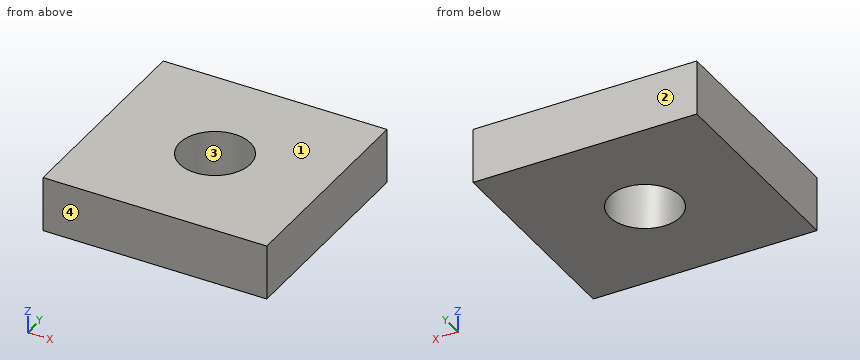
```python
from build123d import *

# Parameters (mm, degrees)
F0_R     = 16.2815755653
F1_DEPTH = 25.4
F3_DEPTH = 25.4


# Not quite as in the source:
# - the program builds the solid bodies; features that only make, move or delete a surface that nothing else refers to are left out


with BuildPart() as f1:
    # F0 (on Top) → F1 (new body)
    with BuildSketch(Plane.XY):
        Polygon((-32.1844741702, 49.3294708431), (-51.5748507939, 49.3294708431), (-51.5748507939, -49.3294708431), (51.5748507939, -49.3294708431), (51.5748507939, 49.3294708431), (-11.7852937953, 49.3294708431), align=None)
        Circle(F0_R, mode=Mode.SUBTRACT)
    extrude(amount=F1_DEPTH)

    # F0 (on Top) → F3 (join)
    with BuildSketch(Plane.XY):
        Polygon((-32.1844741702, 49.3294708431), (-51.5748507939, 49.3294708431), (-51.5748507939, -49.3294708431), (51.5748507939, -49.3294708431), (51.5748507939, 49.3294708431), (-11.7852937953, 49.3294708431), align=None)
        Circle(F0_R, mode=Mode.SUBTRACT)
    extrude(amount=F3_DEPTH)


solid = f1.part
```
The model under review builds one solid part; all positions refer to its coordinate system, in mm. Face numbers are marked on the shaded views. Round coordinates to 2 decimals unless told otherwise and drop trailing zeros. Order: outer loops, then holes, each group sorted by start corner. A loop starts at its lowest first (then second) coordinate and runs counter-clockwise, first axis right, second up. Notation, with made-up numbers: (48, 36.25) -> (104, 36.25) arc R32 ccw to (104, 64.25) -> close; hole circle Ø9 at (46.25, 38). An arc over 180 degrees is marked (long way). One line per item, written item: value. Start each with the question number.
Q1. Wall thickness on line 1 (Y direction, x = 0, z = 10); line 2 (Y direction, x = 3, z = 10.25): over which ranges is each line inside the solid? List them lowest first.
Q2. Take a section at B-B (x = 0). Write out the cut boundary in (y, z), and give its area (3 significant figures).
Q3. Take a section at C-C (z = 22.5). Write out the cut boundary in (x, y), and give its area (3 significant figures).
Q4. Take a section at A-A (y = 0). Write out the cut boundary in (x, z), and give its area (3 significant figures).
Q5. Mouldability with a two-part tool opening along Y and no side actions: class the marked faces 1, 2, 3 and 4 as released by +Y, released by -Y, zero draft, split by the parting line, or undercut.
Reported:
1. line 1: y = -49.33 to -16.28, 16.28 to 49.33
1. line 2: y = -49.33 to -16, 16 to 49.33
2. outline: (-49.33, 0) -> (-16.28, 0) -> (-16.28, 25.4) -> (-49.33, 25.4) -> close; (16.28, 0) -> (49.33, 0) -> (49.33, 25.4) -> (16.28, 25.4) -> close
2. area: 1,680 mm2
3. outline: (-51.57, -49.33) -> (51.57, -49.33) -> (51.57, 49.33) -> (-51.57, 49.33) -> close; hole circle Ø32.56 at (0, 0)
3. area: 9,340 mm2
4. outline: (-51.57, 0) -> (-16.28, 0) -> (-16.28, 25.4) -> (-51.57, 25.4) -> close; (16.28, 0) -> (51.57, 0) -> (51.57, 25.4) -> (16.28, 25.4) -> close
4. area: 1,790 mm2
5. face 1: zero draft
5. face 2: released by +Y
5. face 3: undercut
5. face 4: released by -Y
